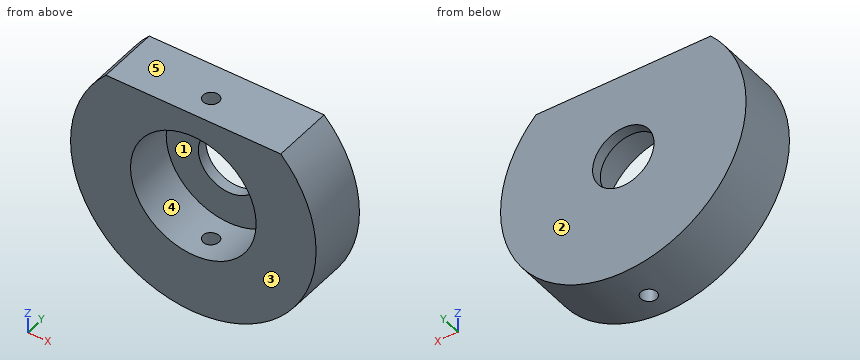
```python
from build123d import *

# Parameters (mm, degrees)
F1_DEPTH = 25.4
F3_R     = 25.9969
F4_DEPTH = 20.9042
F2_R     = 25.9969
F5_DEPTH = 20.9042
F7_D     = 25.4
F7_DEPTH = 21.0058
F7_TIP   = 7.6309298617
F10_D    = 6.5278


with BuildPart() as f1:
    # F0 (on Front) → F1 (new body)
    with BuildSketch(Plane.XZ):
        with BuildLine():
            Line((36.1855936237, 35.6544922009), (-36.1855936237, 35.6544922009))
            ThreePointArc((-36.1855936237, 35.6544922009), (0, -50.8), (36.1855936237, 35.6544922009))
        make_face()
    extrude(amount=F1_DEPTH)

    # F3 (on face) → F4 (join)
    with BuildSketch(Plane.XZ.offset(25.4)):
        Circle(F3_R)
    extrude(amount=-F4_DEPTH)

    # F2 (on face) → F5 (cut)
    with BuildSketch(Plane.XZ.offset(25.4)):
        Circle(F2_R)
    extrude(amount=-F5_DEPTH, mode=Mode.SUBTRACT)

    # F7
    with Locations(Plane.XZ.offset(4.4958)):
        with Locations((0, 0)):
            Hole(F7_D / 2, depth=F7_DEPTH)
            with Locations((0, 0, -(F7_DEPTH + F7_TIP / 2))):  # 118° drill point
                Cone(0, F7_D / 2, F7_TIP, mode=Mode.SUBTRACT)

    # F10 (through all)
    with Locations(Plane.XY.offset(35.6544922009)):
        with Locations((0, -14.9352)):
            Hole(F10_D / 2)


solid = f1.part
```
Geometry check sheet. Reference: the model listing, model coordinates, mm. Face numbers are marked on the shaded views. A direction names the side the tool comes from. Coordinates: 2 decimals unless noted, no trailing zeros. Loops run counter-clockwise (first coordinate to the right, second up) from the corner with the lowest first, then second, coordinate; pieces in that order, holes last. Notation, with made-up numbers: (-29, -7) - (-12, -7) arc R22 cw to (-12, 24) - close; hole circle Ø6 at (17.25, 47.25). An arc over 180 degrees is marked (long way). One line per item, written item: value. Start each with the question number.
(1) Depth check by flat-ended pin: P1, Ø4, axis at y = -20, z = 16, coming from the -X side; P2, Ø23, axis at x = 0, z = 0, coming from the +Y side; P3, Ø1.5, axis at x = 15.5, z = -13.5, coming from the -Y side; P4, Ø8, axis at x = 22.5, y = -11.5, coming from the -Z side. Enter the tip coordinate at first touch or a pass-through.
(2) Cross-section at A-A on z = 0. Enter the section's corners in (x, y), plus the area to 3 significant figures.
(3) Mould release check, pull along Z, two halves, no side actions. Record for the marked faces 3, 4 and 5: released by +Z, released by -Z, zero draft, split by the parting line, or undercut.
(4) Cross-section at B-B on x = 0. Enter the section's corners in (y, z).
(5) Cross-section at D-D on x = -22.5. Enter the section's corners in (y, z), plus the area to 3 significant figures.
(6) Cross-section at C-C on y = -10.5. Enter the section's corners in (x, z), plus the area to 3 significant figures.
(7) Tool access check on the marked faces 1 and 2. Record the directions out of +Z, -Z, +X, -X, +Y, -Y that give a thin tool (end or side, any length) a straight path to the whole face; none if there is none.
(8) Material ranges on line 1 (Y direction, x = 0, z = -31); line 2 (Z direction, x = 0, y = -2.65); line 3 (Y direction, x = -6, z = 15), recorded low to high. Write a range as [from, to].
Results below:
1. P1: stops at x = -48.83
1. P2: passes through
1. P3: stops at y = -4.5
1. P4: stops at z = -47.31
2. outline: (-50.8, -25.4) - (-26, -25.4) - (-26, -4.5) - (-12.7, -4.5) - (-12.7, 0) - (-50.8, 0) - close; (12.7, -4.5) - (26, -4.5) - (26, -25.4) - (50.8, -25.4) - (50.8, 0) - (12.7, 0) - close
2. area: 1,380 mm2
3. face 3: zero draft
3. face 4: undercut
3. face 5: released by +Z
4. outline: (-25.4, -50.8) - (-18.2, -50.8) - (-18.2, -26) - (-25.4, -26) - close; (-25.4, 26) - (-18.2, 26) - (-18.2, 35.65) - (-25.4, 35.65) - close; (-11.67, -50.8) - (0, -50.8) - (0, -12.7) - (-4.5, -12.7) - (-4.5, -26) - (-11.67, -26) - close; (-11.67, 26) - (-4.5, 26) - (-4.5, 12.7) - (0, 12.7) - (0, 35.65) - (-11.67, 35.65) - close
5. outline: (-25.4, -45.55) - (0, -45.55) - (0, 35.65) - (-25.4, 35.65) - (-25.4, 13.02) - (-4.5, 13.02) - (-4.5, -13.02) - (-25.4, -13.02) - close
5. area: 1,520 mm2
6. outline: (-36.19, 35.65) arc R50.8 ccw (long way) to (36.19, 35.65) - close; hole circle Ø51.99 at (0, 0)
6. area: 5,230 mm2
7. face 1: -Y
7. face 2: +Z, -Z, +X, -X, +Y
8. line 1: y = [-25.4, -18.2], [-11.67, 0]
8. line 2: z = [-50.8, -12.7], [12.7, 35.65]
8. line 3: y = [-4.5, 0]
